```python
from build123d import *

# Parameters (mm, degrees)
F0_W     = 101.6
F0_H     = 101.6
F1_DEPTH = 38.1
F3_R     = 6.35
F4_SIZE  = 3.81
F5_T     = -3.175
F2_R     = 6.35
F6_DEPTH = 38.101


with BuildPart() as f1:
    # F0 (on Top) → F1 (new body)
    with BuildSketch(Plane.XY):
        Rectangle(F0_W, F0_H)
    extrude(amount=F1_DEPTH)

    # F3
    f3_edges = [f1.edges().sort_by_distance(p)[0] for p in [
        (-50.8, 50.8, 19.05),
        (50.8, -50.8, 19.05),
        (50.8, 50.8, 19.05),
        (-50.8, -50.8, 19.05),
    ]]
    fillet(f3_edges, radius=F3_R)

    # F4
    f4_edges = [f1.edges().sort_by_distance(p)[0] for p in [
        (0, -50.8, 0),
    ]]
    chamfer(f4_edges, length=F4_SIZE)

    # F5
    f5_openings = [f1.faces().sort_by_distance(p)[0] for p in [
        (0, 0, 38.1),
    ]]
    offset(amount=F5_T, openings=f5_openings)

    # F2 (on face) → F6 (cut, through all)
    with BuildSketch(Plane(origin=(0, 0, 0), x_dir=(1, 0, 0), z_dir=(0, 0, -1))):
        with Locations((-31.430896, 31.430896)):
            Circle(F2_R)
    extrude(amount=-F6_DEPTH, mode=Mode.SUBTRACT)


solid = f1.part
```
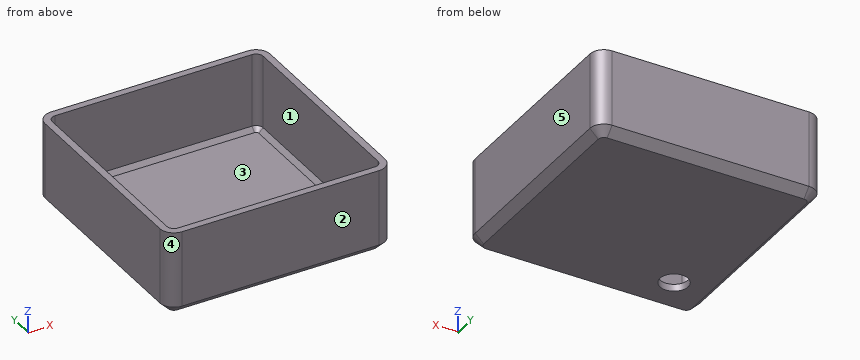
Geometry: final body of the model. Coordinates: model frame, mm. Face numbers are marked on the shaded views. A direction names the side the tool comes from. Round coordinates to 2 decimals unless told otherwise and drop trailing zeros. Loops run counter-clockwise (first coordinate to the right, second up) from the corner with the lowest first, then second, coordinate; pieces in that order, holes last. Notation, with made-up numbers: (53, 70) -> (61, 70) arc R15 cw to (61, 75) -> close; hole circle Ø2 at (-12, 9.5). An arc over 180 degrees is marked (long way). Use one line per item in the form item = value. Start each with the question number.
1) Draft query along Y for the marked faces 3, 4 and 5. Return one class per face: released by +Y, released by -Y, zero draft, split by the parting line, or undercut.
2) First-contact query: P1, Ø10, axis at x = -3, y = 36.5, coming from the +Z side (3 decimals). Flat tip, straight axial feed; report the tip coordinate or a pass-through.
3) Section B-B on y = -7.5. Output: boundary loops of the cut face in (x, z) (3 decimals).
4) Section A-A on z = 28.5. Output: boundary loops of the cut face in (x, y) (3 decimals), then the cut area to 3 significant figures.
5) Line query: L1, parallel to Y at x = 35.5, z = 34 (3 decimals); L2, parallel to X at y = -47, z = 10. Output: solid intervals per line, ascending.
6) Access query for the marked faces 1 and 2. Directions: +Z, -Z, +X, -X, +Y, -Y. A direction counts if a zero-diameter tool reaches every point of the face in a straight line with its end or side. Return the directions, or none.
7) Section D-D on y = -34. Output: boundary loops of the cut face in (x, z) (3 decimals), then the cut area to 3 significant figures.
Response:
q1.face_3 = undercut
q1.face_4 = released by -Y
q1.face_5 = zero draft
q2.P1 = 3.175
q3.outline = (-50.8, 3.81) -> (-46.99, 0) -> (46.99, 0) -> (50.8, 3.81) -> (50.8, 38.1) -> (47.625, 38.1) -> (47.625, 5.125) -> (45.675, 3.175) -> (-45.675, 3.175) -> (-47.625, 5.125) -> (-47.625, 38.1) -> (-50.8, 38.1) -> close
q4.outline = (-50.8, -44.45) arc R6.35 ccw to (-44.45, -50.8) -> (44.45, -50.8) arc R6.35 ccw to (50.8, -44.45) -> (50.8, 44.45) arc R6.35 ccw to (44.45, 50.8) -> (-44.45, 50.8) arc R6.35 ccw to (-50.8, 44.45) -> close; hole (-47.625, -44.45) arc R3.175 ccw to (-44.45, -47.625) -> (44.45, -47.625) arc R3.175 ccw to (47.625, -44.45) -> (47.625, 44.45) arc R3.175 ccw to (44.45, 47.625) -> (-44.45, 47.625) arc R3.175 ccw to (-47.625, 44.45) -> close
q4.area = 1,220 mm^2
q5.L1 = -50.8 to -47.625, 47.625 to 50.8
q5.L2 = -50.27 to -46.34, 46.34 to 50.27
q6.face_1 = +Z
q6.face_2 = +Z, -Z, +X, -X, -Y
q7.outline = (-50.8, 3.81) -> (-46.99, 0) -> (-37.238, 0) -> (-37.238, 3.175) -> (-45.675, 3.175) -> (-47.625, 5.125) -> (-47.625, 38.1) -> (-50.8, 38.1) -> close; (-25.624, 0) -> (46.99, 0) -> (50.8, 3.81) -> (50.8, 38.1) -> (47.625, 38.1) -> (47.625, 5.125) -> (45.675, 3.175) -> (-25.624, 3.175) -> close
q7.area = 497 mm^2
